from build123d import *

# Parameters (mm, degrees)
SKETCH1_R               = 29.5
SKETCH1_R_2             = 5
SKETCH1_R_3             = 2.6
BOSS_EXTRUDE1_DEPTH     = 4
SKETCH1_3_R             = 10
SKETCH1_3_R_2           = 5
BOSS_EXTRUDE2_DEPTH     = 20
CUT_EXTRUDE1_DEPTH      = 47.265537931
CUT_EXTRUDE1_DEPTH_BACK = 47.265537931
SKETCH2_R               = 2


with BuildPart() as part:
    # Sketch1 → Boss-Extrude1 (new body)
    with BuildSketch(Plane(origin=(0, 0, 0), x_dir=(1, 0, 0), z_dir=(0, 1, 0))):
        with Locations(Location((0, 0, 0), (0, 0, 270))):
            Circle(SKETCH1_R)
        with Locations(Location((0, 0, 0), (0, 0, 270))):
            Circle(SKETCH1_R_2, mode=Mode.SUBTRACT)
        with Locations(Location((23.5, 0, 0), (0, 0, 270))):
            Circle(SKETCH1_R_3, mode=Mode.SUBTRACT)
        with Locations(Location((11.75, -20.351596989, 0), (0, 0, 270))):
            Circle(SKETCH1_R_3, mode=Mode.SUBTRACT)
        with Locations(Location((-11.75, -20.351596989, 0), (0, 0, 270))):
            Circle(SKETCH1_R_3, mode=Mode.SUBTRACT)
        with Locations(Location((-23.5, 0, 0), (0, 0, 270))):
            Circle(SKETCH1_R_3, mode=Mode.SUBTRACT)
        with Locations(Location((-11.75, 20.351596989, 0), (0, 0, 270))):
            Circle(SKETCH1_R_3, mode=Mode.SUBTRACT)
        with Locations(Location((11.75, 20.351596989, 0), (0, 0, 270))):
            Circle(SKETCH1_R_3, mode=Mode.SUBTRACT)
    extrude(amount=BOSS_EXTRUDE1_DEPTH)

    # Sketch1_3 → Boss-Extrude2 (add)
    with BuildSketch(Plane(origin=(0, 0, 0), x_dir=(1, 0, 0), z_dir=(0, 1, 0))):
        with Locations(Location((0, 0, 0), (0, 0, 270))):
            Circle(SKETCH1_3_R)
        with Locations(Location((0, 0, 0), (0, 0, 270))):
            Circle(SKETCH1_3_R_2, mode=Mode.SUBTRACT)
    extrude(amount=BOSS_EXTRUDE2_DEPTH)

    # Sketch2 → Cut-Extrude1 (cut, two sides: drawn at the far end of the back side and taken through both)
    with BuildSketch(Plane.XY.offset(-CUT_EXTRUDE1_DEPTH_BACK)):
        with Locations((0, 12)):
            Circle(SKETCH2_R)
    extrude(amount=CUT_EXTRUDE1_DEPTH + CUT_EXTRUDE1_DEPTH_BACK, mode=Mode.SUBTRACT)


solid = part.part
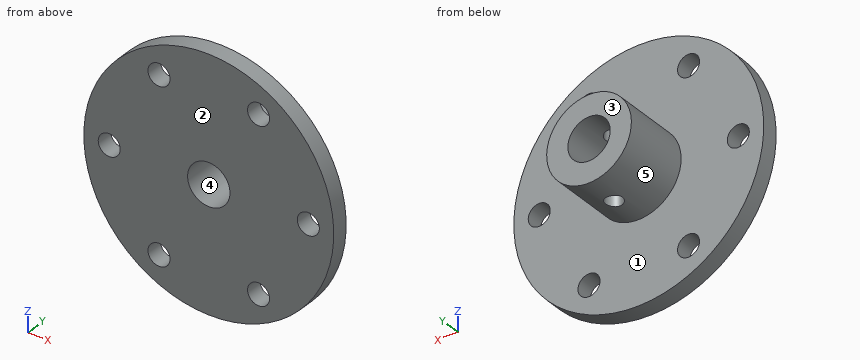
The listing builds one solid part. Answer for the finished solid, in the listing's coordinates (mm). Face numbers are marked on the shaded views. A direction names the side the tool comes from. Give positions to 0.01 mm unless a question says otherwise; leave off trailing zeros. Write each loop counter-clockwise with the first axis right and the second up, starting at its lowest first coordinate (ties: lowest second). Pieces come first, ordered by that corner, then holes.
Item 1: Section C-C, the plane z = -21 is taken. Write down the section's boundary in (x, y), plus the area to 3 significant figures.
Item 2: Section D-D, the plane y = 16.5 is taken. Write down the section's boundary in (x, z), plus the area to 3 significant figures.
Item 3: Section B-B, the plane z = 0 is taken. Write down the section's boundary in (x, y), plus the area to 3 significant figures.
Item 4: Which of the six approach directions +Z, -Z, +X, -X, +Y, -Y give full straight-line access (tool end or side, diameter ignored) to the marked faces 1 and 2?
Item 5: Flat-ended cylindrical pins translate along their axes: P1, Ø12, axis at x = -4, y = 12, coming from the +Z side; P2, Ø6, axis at y = 4, z = 22.5, coming from the -X side; P3, Ø5, axis at x = 12.5, z = -10, coming from the +Y side; P4, Ø3, axis at x = -11.75, z = -20.35, coming from the -Y side. Find the tip coordinate at first contact, or state that the pin passes through.
Item 6: Find the intervals of material crossed by line 1 along X through (y, z) = (2.1, 0); line 2 along X through (y, z) = (15.25, 0); line 3 along Y through (x, z) = (22, 4), in increasing order.
Item 7: Determine the mould class of the marked faces 3, 4 and 5 for opening direction Z: released by +Z, released by -Z, zero draft, split by the parting line, or undercut.
Item 8: Section A-A, the plane x = 0 is taken. Write down the section's boundary in (y, z), plus the area to 3 significant figures.
Completed:
1. outline: (-20.72, 0) - (-14.27, 0) - (-14.27, 4) - (-20.72, 4) - close; (-9.23, 0) - (9.23, 0) - (9.23, 4) - (-9.23, 4) - close; (14.27, 0) - (20.72, 0) - (20.72, 4) - (14.27, 4) - close
1. area: 125 mm2
2. outline: circle Ø20 at (0, 0); hole circle Ø10 at (0, 0)
2. area: 236 mm2
3. outline: (-29.5, 0) - (-26.1, 0) - (-26.1, 4) - (-29.5, 4) - close; (-20.9, 0) - (-5, 0) - (-5, 20) - (-10, 20) - (-10, 4) - (-20.9, 4) - close; (5, 0) - (20.9, 0) - (20.9, 4) - (10, 4) - (10, 20) - (5, 20) - close; (26.1, 0) - (29.5, 0) - (29.5, 4) - (26.1, 4) - close
3. area: 314 mm2
4. face 1: +Y
4. face 2: +Z, -Z, +X, -X, -Y
5. P1: stops at z = 10
5. P2: stops at x = -22.14
5. P3: stops at y = 4
5. P4: passes through
6. line 1: x = -29.5 to -26.1, -20.9 to -5, 5 to 20.9, 26.1 to 29.5
6. line 2: x = -10 to -5, 5 to 10
6. line 3: y = 0 to 4
7. face 3: zero draft
7. face 4: undercut
7. face 5: split by the parting line
8. outline: (0, -29.5) - (4, -29.5) - (4, -10) - (10, -10) - (10, -5) - (0, -5) - close; (0, 5) - (10, 5) - (10, 10) - (4, 10) - (4, 29.5) - (0, 29.5) - close; (14, -10) - (20, -10) - (20, -5) - (14, -5) - close; (14, 5) - (20, 5) - (20, 10) - (14, 10) - close
8. area: 316 mm2
